Verification items for the finished model (mm, model axes). Face numbers are marked on the shaded views. A direction names the side the tool comes from. Coordinates: 2 decimals unless noted, no trailing zeros. Write each loop counter-clockwise with the first axis right and the second up, starting at its lowest first coordinate (ties: lowest second). Pieces come first, ordered by that corner, then holes. Notation, with made-up numbers: (-24, 34) -> (27, 34) arc R18 ccw to (27, 60) -> close; hole circle Ø1 at (39, -0.5). An arc over 180 degrees is marked (long way). Use CSV: the item, a comma, the result in double quotes.
Autodesk Inventor part; units mm, degrees
ref_plane "YZ Plane" through (0, 0, 0) normal (1, 0, 0) x (0, 1, 0)
ref_plane "XZ Plane" through (0, 0, 0) normal (0, 1, 0) x (-1, 0, 0)
ref_plane "XY Plane" through (0, 0, 0) normal (0, 0, 1) x (1, 0, 0)
sketch "Sketch1" plane through (0, 0, 0) normal (0, 1, 0) x (-1, 0, 0)
  circle A0 centre (0, 0) radius 10
  dimension "d0" = 20
extrude "Extrusion1" add sketch "Sketch1" along normal blind 25.5
sketch "Sketch2" plane through (0, 0, 0) normal (0, -1, 0) x (1, 0, 0)
  circle A0 centre (0, 0) radius 6.1
  dimension "d3" = 12.2
extrude "Extrusion2" cut sketch "Sketch2" against normal through all
sketch "Sketch3" plane through (0, 0, 0) normal (0, -1, 0) x (1, 0, 0)
  circle A0 centre (0, 0) radius 10
  circle A1 centre (0, 0) radius 12.5
  dimension "d6" = 25
extrude "Extrusion3" add sketch "Sketch3" against normal blind 5
fillet "Fillet1" radius 2 1 edges at (10, 25.5, 0)
properties part number "Bushing_stempel" material "Brass, Soft Yellow"
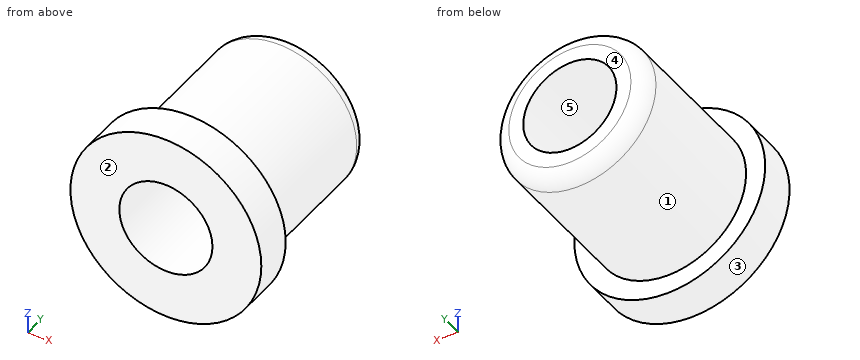
1) Mould release check, pull along X, two halves, no side actions. Record for the marked faces 3, 4 and 5: released by +X, released by -X, zero draft, split by the parting line, or undercut.
Return value:
face 3,"split by the parting line"
face 4,"zero draft"
face 5,"undercut"
2) Cross-section at C-C (y = 2). Record the boundary of the cut face in (x, z), plus the area to 3 significant figures.
Return value:
outline,"circle Ø25 at (0, 0); hole circle Ø12.2 at (0, 0)"
area,"374 mm2"
3) Set-up check for the marked faces 1 and 2: record each of +Z, -Z, +X, -X, +Y, -Y from which the full face is reachable in a straight line by a thin tool's end or side.
Return value:
face 1,"+Y"
face 2,"+Z, -Z, +X, -X, -Y"
4) Cross-section at A-A (z = 0). Record the boundary of the cut face in (x, y).
Return value:
outline,"(-12.5, 0) -> (-6.1, 0) -> (-6.1, 25.5) -> (-8, 25.5) arc R2 ccw to (-10, 23.5) -> (-10, 5) -> (-12.5, 5) -> close; (6.1, 0) -> (12.5, 0) -> (12.5, 5) -> (10, 5) -> (10, 23.5) arc R2 ccw to (8, 25.5) -> (6.1, 25.5) -> close"
5) Gauge pin test, flat ends, axial feed: pin 1 (12 mm diameter, centred on x = 4.5, y = 12, fed in from +Z); pin 2 (1.5 mm diameter, centred on y = 4, z = 5.5, fed in from -X); pin 3 (1.5 mm diameter, centred on x = 2.5, y = 21, fed in from -Z). Record the tip position at first contact, or that the pin passes through.
Return value:
pin 1,"z = 10"
pin 2,"x = -11.56"
pin 3,"z = -9.85"
6) Cross-section at D-D (y = 12). Record the boundary of the cut face in (x, z), plus the area to 3 significant figures.
Return value:
outline,"circle Ø20 at (0, 0); hole circle Ø12.2 at (0, 0)"
area,"197 mm2"
7) Scan lines: L1, parallel to Z at x = 0, y = 20.5; L2, parallel to X at y = 9, z = 0.25; L3, parallel to Y at x = -9.75, z = -7.5. Record each from-to range of solid material in increasing order.
Return value:
L1,"-10 to -6.1, 6.1 to 10"
L2,"-10 to -6.09, 6.09 to 10"
L3,"0 to 5"
8) Cross-section at B-B (x = 0). Record the boundary of the cut face in (y, z).
Return value:
outline,"(0, -12.5) -> (5, -12.5) -> (5, -10) -> (23.5, -10) arc R2 ccw to (25.5, -8) -> (25.5, -6.1) -> (0, -6.1) -> close; (0, 6.1) -> (25.5, 6.1) -> (25.5, 8) arc R2 ccw to (23.5, 10) -> (5, 10) -> (5, 12.5) -> (0, 12.5) -> close"
